Source: CAD feature listing. Evaluate the final solid. Frame: model axes, mm. Face numbers are marked on the shaded views. Coordinates: 2 decimals unless noted, no trailing zeros. Order: outer loops, then holes, each group sorted by start corner. A loop starts at its lowest first (then second) coordinate and runs counter-clockwise, first axis right, second up.
```python
from build123d import *

# Parameters (mm, degrees)
BOSS_EXTRUDE1_DEPTH = 52
CUT_EXTRUDE_1_REACH = 133.119
SKETCH_2_R          = 1.5


with BuildPart() as part:
    # Sketch1 → Boss-Extrude1 (new, symmetric)
    with BuildSketch(Plane.XY):
        with BuildLine():
            Line((-50.530004832, 0), (-50.530004832, 3))
            Line((-50.530004832, 3), (-20.530004832, 3))
            ThreePointArc((-20.530004832, 3), (-12.668388321, 6.819790793), (-10.812717884, 15.361002831))
            Line((-10.812717884, 15.361002831), (-33.559523327, 108.981066609))
            Line((-33.559523327, 108.981066609), (-30.737861628, 110))
            Line((-30.737861628, 110), (-7.014578577, 12.361002831))
            ThreePointArc((-7.014578577, 12.361002831), (-8.870249014, 3.819790793), (-16.731865525, 0))
            Line((-16.731865525, 0), (-50.530004832, 0))
        make_face()
    extrude(amount=BOSS_EXTRUDE1_DEPTH, both=True)

    # Эскиз2 → Вырез-Вытянуть1 (cut, up to next)
    with BuildSketch(Plane(origin=(-3.787634246, -0.920279007, 0), x_dir=(0, 0, -1), z_dir=(0.9717286948053453, 0.2361002831254127, 0)), mode=Mode.PRIVATE) as cut_extrude_1_sk1:
        with Locations(Location((-42, 104.147374262, 0), (0, 0, 90))):
            Circle(SKETCH_2_R)
    cut_extrude_1_tool1 = extrude(cut_extrude_1_sk1.sketch, amount=-CUT_EXTRUDE_1_REACH, mode=Mode.PRIVATE) & part.part
    # Эскиз2 → Вырез-Вытянуть1 (cut, up to next)
    with BuildSketch(Plane(origin=(-3.787634246, -0.920279007, 0), x_dir=(0, 0, -1), z_dir=(0.9717286948053453, 0.2361002831254127, 0)), mode=Mode.PRIVATE) as cut_extrude_1_sk2:
        with Locations(Location((42, 104.147374262, 0), (0, 0, 90))):
            Circle(SKETCH_2_R)
    cut_extrude_1_tool2 = extrude(cut_extrude_1_sk2.sketch, amount=-CUT_EXTRUDE_1_REACH, mode=Mode.PRIVATE) & part.part
    # Эскиз2 → Вырез-Вытянуть1 (cut, up to next)
    with BuildSketch(Plane(origin=(-3.787634246, -0.920279007, 0), x_dir=(0, 0, -1), z_dir=(0.9717286948053453, 0.2361002831254127, 0)), mode=Mode.PRIVATE) as cut_extrude_1_sk3:
        with Locations(Location((42, 34.147374262, 0), (0, 0, 90))):
            Circle(SKETCH_2_R)
    cut_extrude_1_tool3 = extrude(cut_extrude_1_sk3.sketch, amount=-CUT_EXTRUDE_1_REACH, mode=Mode.PRIVATE) & part.part
    # Эскиз2 → Вырез-Вытянуть1 (cut, up to next)
    with BuildSketch(Plane(origin=(-3.787634246, -0.920279007, 0), x_dir=(0, 0, -1), z_dir=(0.9717286948053453, 0.2361002831254127, 0)), mode=Mode.PRIVATE) as cut_extrude_1_sk4:
        with Locations(Location((-42, 34.147374262, 0), (0, 0, 90))):
            Circle(SKETCH_2_R)
    cut_extrude_1_tool4 = extrude(cut_extrude_1_sk4.sketch, amount=-CUT_EXTRUDE_1_REACH, mode=Mode.PRIVATE) & part.part
    add(cut_extrude_1_tool1.solids().sort_by_distance((-28.376859, 100.282713, 42))[0], mode=Mode.SUBTRACT)
    add(cut_extrude_1_tool2.solids().sort_by_distance((-28.376859, 100.282713, -42))[0], mode=Mode.SUBTRACT)
    add(cut_extrude_1_tool3.solids().sort_by_distance((-11.849839, 32.261704, -42))[0], mode=Mode.SUBTRACT)
    add(cut_extrude_1_tool4.solids().sort_by_distance((-11.849839, 32.261704, 42))[0], mode=Mode.SUBTRACT)


solid = part.part
```
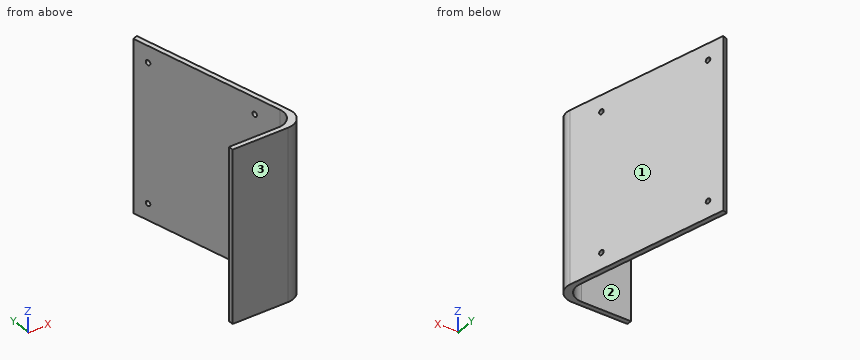
Q1. Section query D-D on x = -44. Output: boundary loops of the cut face in (y, z).
Solutions:
outline: (0, -52) - (3, -52) - (3, 52) - (0, 52) - close
Q2. Section query B-B on x = -25. Output: boundary loops of the cut face in (y, z), plus the area to 3 significant figures.
Solutions:
outline: (0, -52) - (3, -52) - (3, 52) - (0, 52) - close; (73.75, -52) - (86.38, -52) - (86.38, 52) - (73.75, 52) - close
area: 1,630 mm2
Q3. Section query C-C on x = -13.5. Give the number of separate pieces and of enclosed holes in the cut face, plus the area to 3 significant figures.
Solutions:
separate pieces: 2
enclosed holes: 2
area: 1,860 mm2
Q4. Pin query (flat end, axial travel): P1, Ø4, axis at x = -44.5, z = -31.5, coming from the +Y side; P2, Ø10, axis at y = 81.5, z = 14, coming from the -X side; P3, Ø3, axis at y = 74.5, z = -19, coming from the -X side. Return the tip coordinate at first contact, or that it passes through.
Solutions:
P1: stops at y = 3
P2: stops at x = -28.1
P3: stops at x = -25.55
Q5. Material intervals for line 1 along Y through (x, z) = (-45.5, 44); line 2 along X through (y, z) = (51.5, -39); line 3 along X through (y, z) = (103.5, -11.5), sorted ascending.
Solutions:
line 1: y = 0 to 3
line 2: x = -19.59 to -16.52
line 3: x = -32.23 to -29.16
Q6. Pull-direction query (Y, two-part tool) for the marked faces 1, 2 and 3; classes: pulls with the +Y half, pulls with the -Y half, needs draft (parallel to the pull), parting line crosses it, or undercut.
Solutions:
face 1: pulls with the +Y half
face 2: undercut
face 3: pulls with the -Y half
Q7. Section query A-A on z = -33. Output: boundary loops of the cut face in (x, y).
Solutions:
outline: (-50.53, 0) - (-16.73, 0) arc R10 ccw to (-7.01, 12.36) - (-30.74, 110) - (-33.56, 108.98) - (-10.81, 15.36) arc R10 cw to (-20.53, 3) - (-50.53, 3) - close
